Input: part model. Units: mm. Frame: model coordinates. Face numbers are marked on the shaded views. A direction names the side the tool comes from. Round coordinates to 2 decimals unless told otherwise and drop trailing zeros. Order: outer loops, then holes, each group sorted by start corner. A loop starts at its lowest first (then second) coordinate and runs counter-clockwise, first axis right, second up.
Item 1: Cut plane D-D on y = 50.5. Output: boundary loops of the cut face in (x, z).
Item 2: Mould query, pull axis Z, two halves, no side actions, for the marked faces 1, 2 and 3. Classes: released by +Z, released by -Z, zero draft, split by the parting line, or undercut.
Item 3: Cut plane C-C on z = 12.5. Output: boundary loops of the cut face in (x, y), then the cut area to 3 significant figures.
Item 4: First-contact query: pin 1 (3 mm diameter, centred on y = 14, z = -10.5, fed in from -X); pin 2 (10 mm diameter, centred on x = 53, y = 13, fed in from +Z); pin 3 (8.5 mm diameter, centred on x = 13, y = 6.5, fed in from +Z); pin 4 (12 mm diameter, centred on x = -11.5, y = -1.5, fed in from -Z). Flat tips, straight axial feed; report the tip coordinate or a pass-through.
Item 5: Line query: L1, parallel to Y at x = 29, z = 1; L2, parallel to Z at x = 0, y = 49; L3, parallel to Z at x = 48, y = 0. Output: solid intervals per line, ascending.
Item 6: Cut plane B-B on x = -7. Output: boundary loops of the cut face in (y, z), then the cut area to 3 significant figures.
Item 7: Cut plane A-A on y = -12.5. Output: boundary loops of the cut face in (x, z).
Item 8: Reachability of the marked faces 4 and 5 from +Z, -Z, +X, -X, +Y, -Y: full face, straight path, thin tool, end or side. Return the list, or none.
```python
from build123d import *

# Parameters (mm, degrees)
SKETCH_R        = 29.15
PAD_DEPTH       = 58
SKETCH001_R     = 29.15
PAD001_DEPTH    = 68
SKETCH002_R     = 29.15
PAD002_DEPTH    = 68
SKETCH003_R     = 24.15
POCKET_DEPTH    = 58
SKETCH004_R     = 24.15
POCKET001_DEPTH = 68
SKETCH005_R     = 24.15
POCKET002_DEPTH = 68


with BuildPart() as part:
    # Sketch → Pad (new body)
    with BuildSketch(Plane.XY.offset(29.15)):
        Circle(SKETCH_R)
    extrude(amount=-PAD_DEPTH)

    # Sketch001 → Pad001 (join)
    with BuildSketch(Plane.XZ.offset(-68)):
        Circle(SKETCH001_R)
    extrude(amount=PAD001_DEPTH)

    # Sketch002 → Pad002 (join)
    with BuildSketch(Plane.YZ.offset(68)):
        Circle(SKETCH002_R)
    extrude(amount=-PAD002_DEPTH)

    # Sketch003 (on Face5 of Pad002) → Pocket (cut)
    with BuildSketch(Plane.XY.offset(29.15)):
        Circle(SKETCH003_R)
    extrude(amount=-POCKET_DEPTH, mode=Mode.SUBTRACT)

    # Sketch004 (on Face15 of Pocket) → Pocket001 (cut)
    with BuildSketch(Plane(origin=(68, 0, 29.15), x_dir=(0, 1, 0), z_dir=(1, 0, 0))):
        with Locations((0, -29.259423)):
            Circle(SKETCH004_R)
    extrude(amount=-POCKET001_DEPTH, mode=Mode.SUBTRACT)

    # Sketch005 (on Face7 of Pocket001) → Pocket002 (cut)
    with BuildSketch(Plane(origin=(0, 68, 29.15), x_dir=(-1, 0, 0), z_dir=(0, 1, 0))):
        with Locations((0, -28.95468)):
            Circle(SKETCH005_R)
    extrude(amount=-POCKET002_DEPTH, mode=Mode.SUBTRACT)


solid = part.part
```
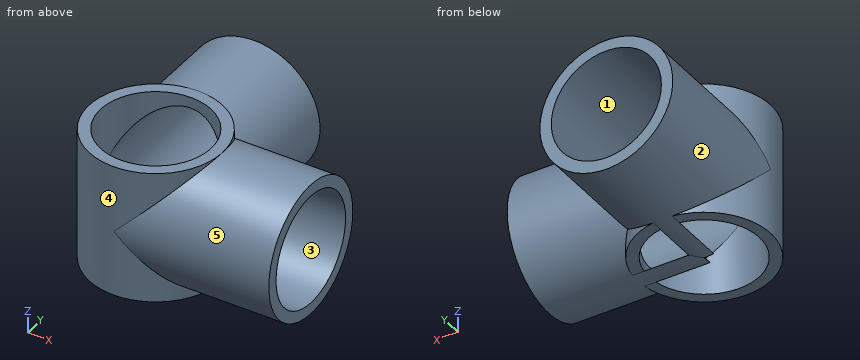
From the geometry:
1. outline: circle Ø58.3 at (0, 0); hole circle Ø48.3 at (0, 0.2)
2. face 1: undercut
2. face 2: split by the parting line
2. face 3: undercut
3. outline: (-26.33, 12.5) arc R29.15 ccw to (12.5, -26.33) - (68, -26.33) - (68, -20.6) - (12.61, -20.6) arc R24.15 cw to (-20.78, 12.3) - (-20.78, 68) - (-26.33, 68) - close; (20.78, 20.6) - (68, 20.6) - (68, 26.33) - (26.33, 26.33) - (26.33, 68) - (20.78, 68) - close
3. area: 1,470 mm2
4. pin 1: stops at x = -27.73
4. pin 2: stops at z = 28.03
4. pin 3: stops at z = -28.85
4. pin 4: passes through
5. L1: y = -29.13 to -24.12, 24.12 to 68
5. L2: z = -29.15 to -23.95, 24.35 to 29.15
5. L3: z = -29.15 to -24.26, 24.04 to 29.15
6. outline: (-28.3, -28.85) - (-23.11, -28.85) - (-23.11, 29.15) - (-28.3, 29.15) - close; (23.11, -28.85) - (28.3, -28.85) - (28.3, -28.3) - (68, -28.3) - (68, -22.92) - (23.11, -22.92) - close; (23.11, 23.31) - (68, 23.31) - (68, 28.3) - (28.3, 28.3) - (28.3, 29.15) - (23.11, 29.15) - close
6. area: 773 mm2
7. outline: (-26.33, -28.85) - (-20.66, -28.85) - (-20.66, 29.15) - (-26.33, 29.15) - close; (20.66, -28.85) - (26.33, -28.85) - (26.33, -26.33) - (68, -26.33) - (68, -20.77) - (20.66, -20.77) - close; (20.66, 20.55) - (68, 20.55) - (68, 26.33) - (26.33, 26.33) - (26.33, 29.15) - (20.66, 29.15) - close
8. face 4: none
8. face 5: +X
